Could you check a few things on this model? Use its own coordinates, in mm. A direction names the side the tool comes from. Round coordinates to 2 decimals unless told otherwise and drop trailing zeros. Loops run counter-clockwise (first coordinate to the right, second up) from the corner with the lowest first, then second, coordinate; pieces in that order, holes last. Notation, with made-up numbers: (51.25, 57) -> (110.25, 57) arc R26 ccw to (110.25, 79) -> close; hole circle Ø2 at (28, -7.5). An arc over 180 degrees is marked (long way). Write each question's results on one line, items separated by ' | '.
from build123d import *

# Parameters (mm, degrees)
SKETCH1_W                    = 8
SKETCH1_H                    = 8
BOSS_EXTRUDE1_DEPTH          = 7
SKETCH3_R                    = 39.5
CUT_EXTRUDE1_DEPTH           = 6
SKETCH5_R                    = 2.25
SKETCH5_R_2                  = 1.6
BOSS_EXTRUDE2_DEPTH          = 6
CHAMFER1_SIZE                = 2.5
CIRPATTERN1_COUNT            = 4
CHAMFER1_OF_CIRPATTERN1_SIZE = 2.5
SKETCH4_R                    = 12.5
CUT_EXTRUDE2_DEPTH           = 77.602872009
CUT_EXTRUDE2_DEPTH_BACK      = 77.602872009
M3X0_5_TAPPED_HOLE1_D        = 2.5
CHAMFER2_SIZE                = 1
FILLET1_R                    = 2.5
SKETCH8_R                    = 1.6
CUT_EXTRUDE3_DEPTH           = 77.602872009


with BuildPart() as part:
    # Sketch1 → Boss-Extrude1 (new body)
    with BuildSketch(Plane(origin=(0, 0, 0), x_dir=(1, 0, 0), z_dir=(0, 1, 0))):
        with BuildLine():
            Line((4, 41.306779105), (4, 50))
            ThreePointArc((4, 50), (0, 54), (-4, 50))
            Line((-4, 50), (-4, 41.306779105))
            ThreePointArc((-4, 41.306779105), (0, 41.5), (4, 41.306779105))
        make_face()
        with BuildLine():
            Line((50, 4), (41.306779105, 4))
            ThreePointArc((41.306779105, 4), (41.45166663, 2.002332035), (41.5, 0))
            ThreePointArc((41.5, 0), (41.45166663, -2.002332035), (41.306779105, -4))
            Line((41.306779105, -4), (50, -4))
            ThreePointArc((50, -4), (54, 0), (50, 4))
        make_face()
        with BuildLine():
            ThreePointArc((-41.306779105, -4), (-41.5, 0), (-41.306779105, 4))
            Line((-41.306779105, 4), (-50, 4))
            ThreePointArc((-50, 4), (-54, 0), (-50, -4))
            Line((-50, -4), (-41.306779105, -4))
        make_face()
        with BuildLine():
            Line((4, -50), (4, -41.306779105))
            ThreePointArc((4, -41.306779105), (0, -41.5), (-4, -41.306779105))
            Line((-4, -41.306779105), (-4, -50))
            ThreePointArc((-4, -50), (0, -54), (4, -50))
        make_face()
        with BuildLine():
            Line((41.306779105, -4), (4, -4))
            Line((4, -4), (4, -41.306779105))
            ThreePointArc((4, -41.306779105), (29.344931419, -29.344931419), (41.306779105, -4))
        make_face()
        with BuildLine():
            ThreePointArc((41.306779105, 4), (29.344931419, 29.344931419), (4, 41.306779105))
            Line((4, 41.306779105), (4, 4))
            Line((4, 4), (41.306779105, 4))
        make_face()
        with BuildLine():
            Line((-4, 4), (-4, 41.306779105))
            ThreePointArc((-4, 41.306779105), (-29.344931419, 29.344931419), (-41.306779105, 4))
            Line((-41.306779105, 4), (-4, 4))
        make_face()
        with BuildLine():
            Line((-4, -41.306779105), (-4, -4))
            Line((-4, -4), (-41.306779105, -4))
            ThreePointArc((-41.306779105, -4), (-29.344931419, -29.344931419), (-4, -41.306779105))
        make_face()
        with BuildLine():
            Line((41.306779105, 4), (4, 4))
            Line((4, 4), (4, -4))
            Line((4, -4), (41.306779105, -4))
            ThreePointArc((41.306779105, -4), (41.45166663, -2.002332035), (41.5, 0))
            ThreePointArc((41.5, 0), (41.45166663, 2.002332035), (41.306779105, 4))
        make_face()
        with BuildLine():
            Line((4, 4), (4, 41.306779105))
            ThreePointArc((4, 41.306779105), (0, 41.5), (-4, 41.306779105))
            Line((-4, 41.306779105), (-4, 4))
            Line((-4, 4), (4, 4))
        make_face()
        with BuildLine():
            Line((-4, -4), (-4, 4))
            Line((-4, 4), (-41.306779105, 4))
            ThreePointArc((-41.306779105, 4), (-41.5, 0), (-41.306779105, -4))
            Line((-41.306779105, -4), (-4, -4))
        make_face()
        with BuildLine():
            Line((4, -41.306779105), (4, -4))
            Line((4, -4), (-4, -4))
            Line((-4, -4), (-4, -41.306779105))
            ThreePointArc((-4, -41.306779105), (0, -41.5), (4, -41.306779105))
        make_face()
        Rectangle(SKETCH1_W, SKETCH1_H)
    extrude(amount=BOSS_EXTRUDE1_DEPTH)

    # Sketch3 → Cut-Extrude1 (cut)
    with BuildSketch(Plane(origin=(0, 7, 0), x_dir=(1, 0, 0), z_dir=(0, 1, 0))):
        with Locations(Location((0, 0, 0), (0, 0, 270))):
            Circle(SKETCH3_R)
    extrude(amount=-CUT_EXTRUDE1_DEPTH, mode=Mode.SUBTRACT)

    # Sketch5 → Boss-Extrude2 (add)
    with BuildSketch(Plane(origin=(0, 1, 0), x_dir=(1, 0, 0), z_dir=(0, 1, 0))):
        with Locations(Location((-10.606601718, 10.606601718, 0), (0, 0, 270))):
            Circle(SKETCH5_R)
        with Locations(Location((-10.606601718, 10.606601718, 0), (0, 0, 270))):
            Circle(SKETCH5_R_2, mode=Mode.SUBTRACT)
    boss_extrude2 = extrude(amount=BOSS_EXTRUDE2_DEPTH)

    # Chamfer1
    chamfer1_edges = [part.edges().sort_by_distance(p)[0] for p in [
        (-10.606601718, 1, -12.856601718),
    ]]
    chamfer(chamfer1_edges, length=CHAMFER1_SIZE)

    # CirPattern1: Boss-Extrude2 ×4 about axis
    cirpattern1_axis = Axis((0, 0, 0), (0, 1, 0))
    for i in range(1, CIRPATTERN1_COUNT):
        add(boss_extrude2.rotate(cirpattern1_axis, i * 360 / CIRPATTERN1_COUNT))

    # Chamfer1 of CirPattern1
    chamfer1_of_cirpattern1_edges = [part.edges().sort_by_distance(p)[0] for p in [
        (-12.856601718, 1, 10.606601718),
        (10.606601718, 1, 12.856601718),
        (12.856601718, 1, -10.606601718),
    ]]
    chamfer(chamfer1_of_cirpattern1_edges, length=CHAMFER1_OF_CIRPATTERN1_SIZE)

    # Sketch4 → Cut-Extrude2 (cut, two sides)
    with BuildSketch(Plane(origin=(0, 1, 0), x_dir=(1, 0, 0), z_dir=(0, 1, 0))) as cut_extrude2_sk:
        with Locations(Location((0, 0, 0), (0, 0, 270))):
            Circle(SKETCH4_R)
    extrude(amount=CUT_EXTRUDE2_DEPTH, mode=Mode.SUBTRACT)
    extrude(cut_extrude2_sk.sketch, amount=-CUT_EXTRUDE2_DEPTH_BACK, mode=Mode.SUBTRACT)

    # M3x0.5 Tapped Hole1 (through all)
    with Locations(Plane(origin=(0, 7, 0), x_dir=(1, 0, 0), z_dir=(0, 1, 0))):
        with Locations((0, 50), (50, 0), (-50, 0), (0, -50)):
            Hole(M3X0_5_TAPPED_HOLE1_D / 2)

    # Chamfer2
    chamfer2_edges = [part.edges().sort_by_distance(p)[0] for p in [
        (0, 7, -39.5),
    ]]
    chamfer(chamfer2_edges, length=CHAMFER2_SIZE)

    # Fillet1
    fillet1_edges = [part.edges().sort_by_distance(p)[0] for p in [
        (4, 3.5, 41.306779105),
        (-4, 3.5, 41.306779105),
        (-41.306779105, 3.5, 4),
        (-41.306779105, 3.5, -4),
        (-4, 3.5, -41.306779105),
        (4, 3.5, -41.306779105),
        (41.306779105, 3.5, -4),
        (41.306779105, 3.5, 4),
    ]]
    fillet(fillet1_edges, radius=FILLET1_R)

    # Sketch8 → Cut-Extrude3 (cut, through all)
    with BuildSketch(Plane(origin=(0, 1, 0), x_dir=(1, 0, 0), z_dir=(0, 1, 0))):
        with Locations(Location((10.606601718, 10.606601718, 0), (0, 0, 270))):
            Circle(SKETCH8_R)
        with Locations(Location((-10.606601718, 10.606601718, 0), (0, 0, 270))):
            Circle(SKETCH8_R)
        with Locations(Location((-10.606601718, -10.606601718, 0), (0, 0, 270))):
            Circle(SKETCH8_R)
        with Locations(Location((10.606601718, -10.606601718, 0), (0, 0, 270))):
            Circle(SKETCH8_R)
    extrude(amount=-CUT_EXTRUDE3_DEPTH, mode=Mode.SUBTRACT)


solid = part.part
1) If we mould it in two halves opening along X, with no side actions, what happens to faces 1 (the conical face through (12.488, 3.379, -12.05)), 2 (the flat face through (36, 7, 20)), 3 (the cylindrical face through (-29.61, 3.45, 29.08))? For each: released by +X, released by -X, zero draft, split by the parting line, or undercut.
Model answer:
face 1: undercut | face 2: zero draft | face 3: released by -X
2) I want a section at A-A, the plane z = 0. Write out the boundary of the cut face in (x, y), plus the area to 3 significant figures.
Model answer:
outline: (-54, 0) -> (-51.25, 0) -> (-51.25, 7) -> (-54, 7) -> close; (-48.75, 0) -> (-12.5, 0) -> (-12.5, 1) -> (-39.5, 1) -> (-39.5, 6) -> (-40.5, 7) -> (-48.75, 7) -> close; (12.5, 0) -> (48.75, 0) -> (48.75, 7) -> (40.5, 7) -> (39.5, 6) -> (39.5, 1) -> (12.5, 1) -> close; (51.25, 0) -> (54, 0) -> (54, 7) -> (51.25, 7) -> close | area: 221 mm2
3) I'm going to push flat-ended pins straight in: pin 1 (2 mm diameter, centred on y = 2.5, z = 43, fed in from -X); pin 2 (1 mm diameter, centred on x = 30.5, y = 5.5, fed in from -Z); pin 3 (1.9 mm diameter, centred on y = 4.5, z = -47.5, fed in from -X); pin 4 (2 mm diameter, centred on x = 0, z = 50, fed in from +Y). Where does each tip first touch, or does it pass through?
Model answer:
pin 1: stops at x = -4.51 | pin 2: stops at z = -28.67 | pin 3: stops at x = -4 | pin 4: passes through
4) I want a section at B-B, the plane x = 0. Write out the boundary of the cut face in (y, z), plus the area to 3 significant figures.
Model answer:
outline: (0, -54) -> (7, -54) -> (7, -51.25) -> (0, -51.25) -> close; (0, -48.75) -> (7, -48.75) -> (7, -40.5) -> (6, -39.5) -> (1, -39.5) -> (1, -12.5) -> (0, -12.5) -> close; (0, 12.5) -> (1, 12.5) -> (1, 39.5) -> (6, 39.5) -> (7, 40.5) -> (7, 48.75) -> (0, 48.75) -> close; (0, 51.25) -> (7, 51.25) -> (7, 54) -> (0, 54) -> close | area: 221 mm2
5) For faces 4 (the flat face through (47, 3, -4)), 5 (the flat face through (-4, 3, -47)), 6 (the cylindrical face through (8.53, 5.23, -11.47)), which set-ups out of +Z, -Z, +X, -X, +Y, -Y let a thin tool reach every point of the face, with its end or its side?
Model answer:
face 4: -Z, +X, +Y, -Y | face 5: -Z, -X, +Y, -Y | face 6: +Y
6) I need wall thicknesses on line 1 (X direction, y = 1.5, z = 7); line 2 (X direction, y = 1.75, z = 8); line 3 (X direction, y = 4.5, z = 10). Which ranges of each line are inside material? Lowest first, please.
Model answer:
line 1: x = -40.91 to -38.87, -12.85 to -10.36, 10.36 to 12.85, 38.87 to 40.91 | line 2: x = -40.72 to -38.68, -13.64 to -9.6, 9.6 to 13.64, 38.68 to 40.72 | line 3: x = -40.28 to -38.21, -12.77 to -12.09, -9.13 to -8.44, 8.44 to 9.13, 12.09 to 12.77, 38.21 to 40.28
